Source: three-view drawing plus pictorial views. Frame: mm from the lowest corner of the part. A direction names the side the tool comes from. Give positions to 0.01 mm unless a question says otherwise; leave off trailing zeros. Loops run counter-clockwise (first coordinate to the right, second up) from the corner with the lowest first, then second, coordinate; pieces in that order, holes last.
1. Section A-A, the plane x = 5.25. Output: boundary loops of the cut face in (y, z), then the cut area to 3 significant figures.
2. Section C-C, the plane y = 4.15. Output: boundary loops of the cut face in (x, z), then the cut area to 3 significant figures.
3. Section B-B, the plane z = 4. Output: boundary loops of the cut face in (x, y).
4. First-contact query: P1, Ø2, axis at x = 4.5, z = 4, coming from the -Y side. Flat tip, straight axial feed; report the tip coordinate or a pass-through.
5. Draft query along Z for the marked faces 3, 4, 5 and 6. Return one class per face: +Z half, -Z half, draft (parallel to the pull), parting line (faces both ways), or undercut.
6. Access query for the marked faces 1 and 2. Directions: +Z, -Z, +X, -X, +Y, -Y. A direction counts if a zero-diameter tool reaches every point of the face in a straight line with its end or side. Return the directions, or none.
7. Material intervals for line 1 along X through (y, z) = (4.15, 2); line 2 along Z through (x, y) = (6, 2.15), sorted ascending.
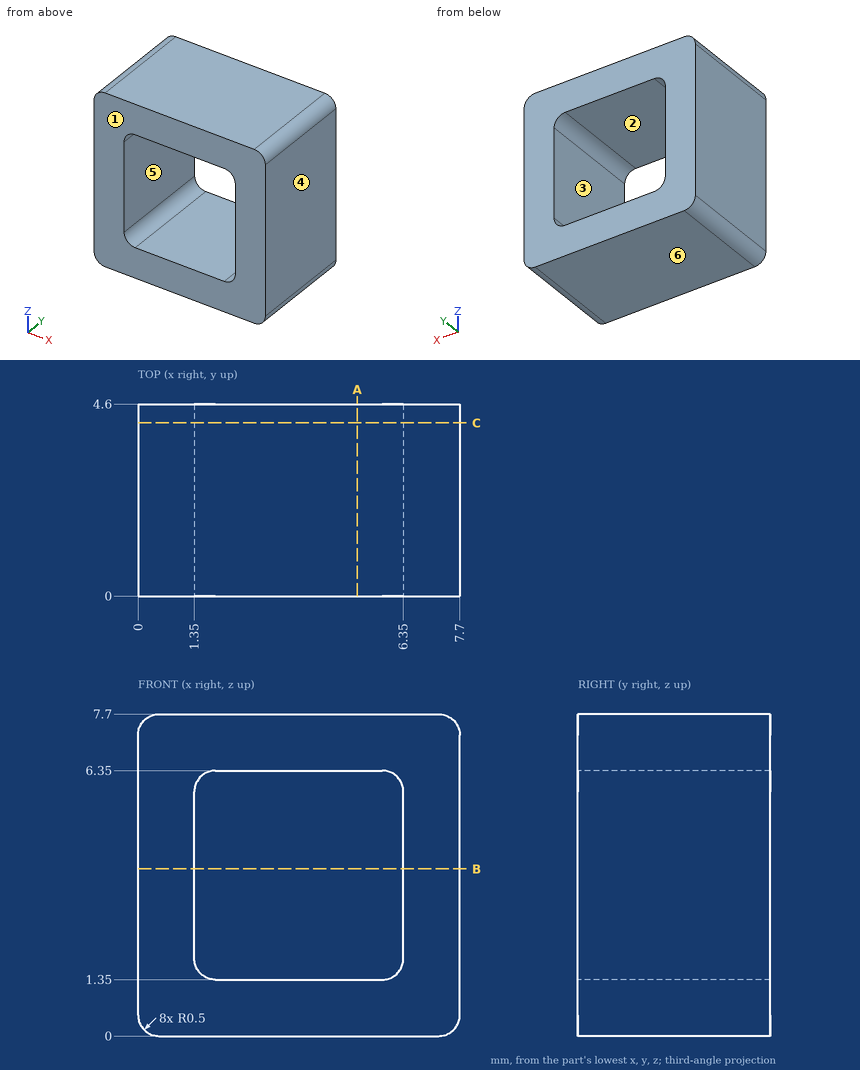
Answers below:
1. outline: (0, 0) - (4.6, 0) - (4.6, 1.35) - (0, 1.35) - close; (0, 6.35) - (4.6, 6.35) - (4.6, 7.7) - (0, 7.7) - close
1. area: 12.4 mm2
2. outline: (0, 0.5) arc R0.5 ccw to (0.5, 0) - (7.2, 0) arc R0.5 ccw to (7.7, 0.5) - (7.7, 7.2) arc R0.5 ccw to (7.2, 7.7) - (0.5, 7.7) arc R0.5 ccw to (0, 7.2) - close; hole (1.35, 1.85) arc R0.5 ccw to (1.85, 1.35) - (5.85, 1.35) arc R0.5 ccw to (6.35, 1.85) - (6.35, 5.85) arc R0.5 ccw to (5.85, 6.35) - (1.85, 6.35) arc R0.5 ccw to (1.35, 5.85) - close
2. area: 34.3 mm2
3. outline: (0, 0) - (1.35, 0) - (1.35, 4.6) - (0, 4.6) - close; (6.35, 0) - (7.7, 0) - (7.7, 4.6) - (6.35, 4.6) - close
4. P1: passes through
5. face 3: undercut
5. face 4: draft
5. face 5: undercut
5. face 6: -Z half
6. face 1: +Z, -Z, +X, -X, -Y
6. face 2: +Y, -Y
7. line 1: x = 0 to 1.35, 6.35 to 7.7
7. line 2: z = 0 to 1.37, 6.33 to 7.7
